```python
from build123d import *

# Parameters (mm, degrees)
SKETCH1_R           = 15
SKETCH1_R_2         = 10
BOSS_EXTRUDE1_DEPTH = 30
SKETCH2_R           = 15
BOSS_EXTRUDE2_DEPTH = 5
SKETCH7_R           = 2.5


with BuildPart() as part:
    # Sketch1 → Boss-Extrude1 (new body)
    with BuildSketch(Plane(origin=(0, 0, 0), x_dir=(1, 0, 0), z_dir=(0, 1, 0))):
        with Locations(Location((0, 0, 0), (0, 0, 270))):  # turned: the seam where the file's is
            Circle(SKETCH1_R)
        with Locations(Location((0, 0, 0), (0, 0, 270))):  # turned: the seam where the file's is
            Circle(SKETCH1_R_2, mode=Mode.SUBTRACT)
    extrude(amount=BOSS_EXTRUDE1_DEPTH)

    # Sketch2 → Boss-Extrude2 (add)
    with BuildSketch(Plane.XZ):
        with Locations(Location((0, 0, 0), (0, 0, 270))):  # turned: the seam where the file's is
            Circle(SKETCH2_R)
    extrude(amount=BOSS_EXTRUDE2_DEPTH)

    # Sweep6: sweep along a path in Sketch3
    with BuildLine(Plane.XY) as sweep6_path:
        Line((15, 25), (19, 25))
        ThreePointArc((19, 25), (31.5, 12.5), (19, 0))
        Line((19, 0), (15, 0))
        Line((15, 0), (15, 25))
    # Sketch7 → Sweep6 (sweep)
    with BuildSketch(Plane(origin=(15, 0, 0), x_dir=(0, 0, -1), z_dir=(1, 0, 0))):
        with Locations((0, 25)):
            Circle(SKETCH7_R)
    sweep(path=sweep6_path.line, transition=Transition.RIGHT)


solid = part.part
```
Check sheet for the modelled part. Datum: model origin and axes. Units: mm. A direction names the side the tool comes from. Round coordinates to 2 decimals unless told otherwise and drop trailing zeros. Order: outer loops, then holes, each group sorted by start corner. A loop starts at its lowest first (then second) coordinate and runs counter-clockwise, first axis right, second up.
1) Section check B-B (x = 0). Record the boundary of the cut face in (y, z).
2) Mould release check, pull along X, two halves, no side actions. Record for faces 4 (the cylindrical face through (-9.76, 14.79, -2.17)), 5 (the cylindrical face through (17.39, 27.48, 0.33)), 6 (the flat face through (-10, 30, 3)): +X half, -X half, draft (parallel to the pull), parting line (faces both ways), or undercut.
3) Go/stop test with flat-tipped pins: pin 1 Ø6 at (x, y) = (28.5, 9.5) entering from -Z; pin 2 Ø12 at (y, z) = (7, -3.5) entering from +X; pin 3 Ø2 at (y, z) = (1.5, -8) entering from +X. Record where each tip stops, or that it passes through.
4) Section check C-C (z = -8). Record the boundary of the cut face in (x, y), and give its area (3 significant figures).
5) Section check A-A (z = 0). Record the boundary of the cut face in (x, y), and give its area (3 significant figures).
6) Scan lines: line 1 (Y direction, x = 2.5, z = 6); line 2 (X direction, y = 18.25, z = 0); line 3 (X direction, y = 21, z = 0). Record each from-to range of solid material in increasing order.
7) Tool access check on faces 1 (the flat face through (0, 0, 0)), 2 (the cylindrical face through (17.33, -2.48, 0.33)), 3 (the flat face through (0, -5, 0)). Record the directions out of +Z, -Z, +X, -X, +Y, -Y that give a thin tool (end or side, any length) a straight path to the whole face; none if there is none.
8) Section check D-D (y = 17). Give the number of separate pieces and of enclosed holes in the cut face, and give its area (3 significant figures).
Result:
1. outline: (-5, -15) - (30, -15) - (30, -10) - (0, -10) - (0, 10) - (30, 10) - (30, 15) - (-5, 15) - close
2. face 4: undercut
2. face 5: undercut
2. face 6: draft
3. pin 1: stops at z = -2.5
3. pin 2: stops at x = 33.99
3. pin 3: stops at x = 13.27
4. outline: (-12.69, -5) - (12.69, -5) - (12.69, 30) - (6, 30) - (6, 0) - (-6, 0) - (-6, 30) - (-12.69, 30) - close
4. area: 528 mm2
5. outline: (-15, -5) - (15, -5) - (15, -2.5) - (19, -2.5) arc R15 ccw to (19, 27.5) - (15, 27.5) - (15, 30) - (10, 30) - (10, 0) - (-10, 0) - (-10, 30) - (-15, 30) - close; hole (17.5, 2.5) - (19, 2.5) arc R10 ccw to (19, 22.5) - (17.5, 22.5) - close
5. area: 736 mm2
6. line 1: y = -5 to 0
6. line 2: x = -15 to -10, 10 to 17.5, 27.18 to 32.85
6. line 3: x = -15 to -10, 10 to 17.5, 24.27 to 31.36
7. face 1: +Y
7. face 2: none
7. face 3: +Z, -Z, +X, -X, -Y
8. separate pieces: 2
8. enclosed holes: 1
8. area: 424 mm2
